Input: dimensioned drawing with shaded views. Units: mm. Origin: part minimum x, y, z. A direction names the side the tool comes from. Round coordinates to 2 decimals unless told otherwise and drop trailing zeros. Loops run counter-clockwise (first coordinate to the right, second up) from the corner with the lowest first, then second, coordinate; pieces in that order, holes last. Notation, with made-up numbers: M 28.25,-38.5 L 64.25,-38.5 A35 ccw 64.25,-2.5 Z; hole C 27.25,31.25 d5. An arc over 180 degrees is marked long. Answer as CSV lines item,"result". Start each with the question number.
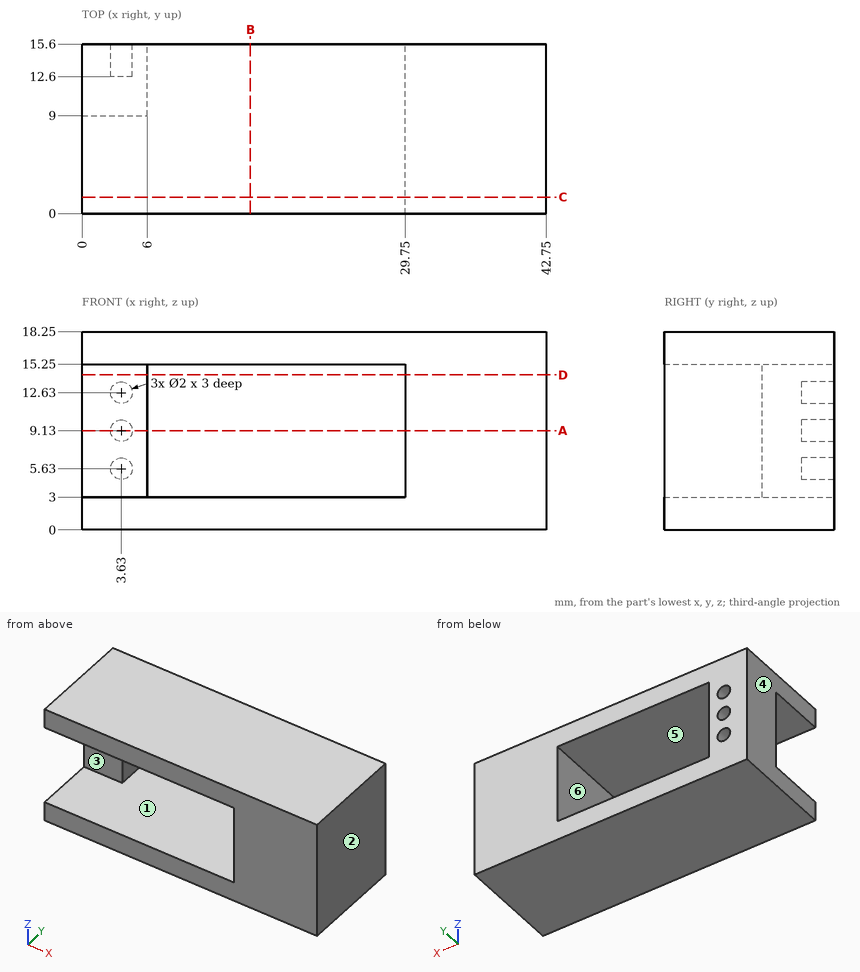
1) Mould query, pull axis X, two halves, no side actions, for the marked faces 1, 2 and 3. Classes: pulls with the +X half, pulls with the -X half, needs draft (parallel to the pull), parting line crosses it, or undercut.
2) Access query for the marked faces 4, 5 and 6. Directions: +Z, -Z, +X, -X, +Y, -Y. A direction counts if a zero-diameter tool reaches every point of the face in a straight line with its end or side. Return the directions, or none.
3) Ray query, line 1 along X through (y, z) = (13.6, 9.13); line 2 along Z through (x, y) = (2, 3); line 3 along X through (y, z) = (3.25, 8.75). Return the intervals inside material, ascending.
4) Section B-B, the plane x = 15.5. Return loops of the section in (y, z).
5) Section A-A, the plane z = 9.13. Return loops of the section in (x, y), and give its area (3 significant figures).
6) Section C-C, the plane y = 1.5. Return loops of the section in (x, z), and give its area (3 significant figures).
7) Section D-D, the plane z = 14.25. Return loops of the section in (x, y), and give its area (3 significant figures).
8) Contact query for flat-ended pins moving along their axis: pin 1 Ø5 at (x, z) = (2.5, 11.5) entering from -Y; pin 2 Ø1.2 at (x, z) = (3.63, 9.13) entering from +Y; pin 3 Ø2 at (y, z) = (5.5, 11.5) entering from -X. Output: stop coordinate, or through.
Findings below:
1,face 1,"undercut"
1,face 2,"pulls with the +X half"
1,face 3,"needs draft"
2,face 4,"+Z, -Z, -X, +Y, -Y"
2,face 5,"-Y"
2,face 6,"+Y, -Y"
3,line 1,"0 to 2.63, 4.63 to 6, 29.75 to 42.75"
3,line 2,"0 to 3, 15.25 to 18.25"
3,line 3,"29.75 to 42.75"
4,outline,"M 0,0 L 15.6,0 L 15.6,3 L 0,3 Z; M 0,15.25 L 15.6,15.25 L 15.6,18.25 L 0,18.25 Z"
5,outline,"M 0,9 L 6,9 L 6,15.6 L 4.63,15.6 L 4.63,12.6 L 2.63,12.6 L 2.63,15.6 L 0,15.6 Z; M 29.75,0 L 42.75,0 L 42.75,15.6 L 29.75,15.6 Z"
5,area,"236 mm²"
6,outline,"M 0,0 L 42.75,0 L 42.75,18.25 L 0,18.25 L 0,15.25 L 29.75,15.25 L 29.75,3 L 0,3 Z"
6,area,"416 mm²"
7,outline,"M 0,9 L 6,9 L 6,15.6 L 0,15.6 Z; M 29.75,0 L 42.75,0 L 42.75,15.6 L 29.75,15.6 Z"
7,area,"242 mm²"
8,pin 1,"y = 9"
8,pin 2,"y = 12.6"
8,pin 3,"x = 29.75"
